CAD build for the part. Positions are in the model's coordinates, mm. Face numbers are marked on the shaded views. A direction names the side the tool comes from. Coordinates: 2 decimals unless noted, no trailing zeros. Loops run counter-clockwise (first coordinate to the right, second up) from the corner with the lowest first, then second, coordinate; pieces in that order, holes last. Notation, with made-up numbers: (-5, 57) -> (26, 57) arc R15 cw to (26, 80) -> close; hole circle Ø5 at (-14.75, 33.5). An arc over 180 degrees is marked (long way). Write each question's results on one line, items separated by ' | '.
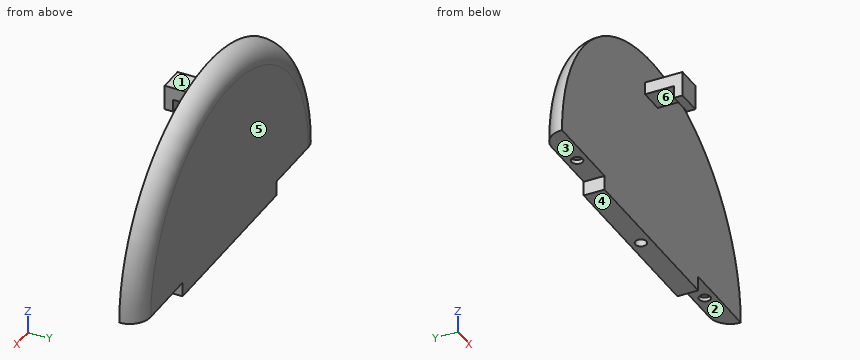
from build123d import *

# Parameters (mm, degrees)
CUT_EXTRUDE1_DEPTH       = 5
CUT_EXTRUDE3_DEPTH       = 45
SKETCH8_R                = 40
CUT_EXTRUDE4_DEPTH       = 32
SKETCH9_R                = 32
SKETCH9_R_2              = 24.5
CUT_EXTRUDE5_DEPTH       = 14
SKETCH10_R               = 26
CUT_EXTRUDE6_DEPTH       = 14
FILLET1_R                = 7
FILLET2_R                = 7
CUT_REVOLVE1_START       = 22
CUT_REVOLVE1_DEPTH       = 30.5
CUT_EXTRUDE12_DEPTH      = 5
SKETCH18_W               = 13
SKETCH18_H               = 8
CUT_EXTRUDE13_DEPTH      = 5
INTERSECT1_OUTLINE_R     = 42
INTERSECT1_DEPTH         = 55
SKETCH20_W               = 6
SKETCH20_H               = 3
BOSS_EXTRUDE1_DEPTH      = 8
BOSS_EXTRUDE2_DEPTH      = 1
BOSS_EXTRUDE2_DEPTH_BACK = 1
SKETCH21_W               = 6
SKETCH21_H               = 6
BOSS_EXTRUDE3_DEPTH      = 7
SKETCH19_R               = 1.35
CUT_EXTRUDE14_DEPTH      = 8
SKETCH23_W               = 20
SKETCH23_H               = 7
CUT_EXTRUDE15_DEPTH      = 7
SKETCH24_W               = 44
SKETCH24_H               = 3.5
CUT_EXTRUDE16_DEPTH      = 5


with BuildPart() as part:
    # Sketch1 → Revolve1 (revolve)
    with BuildSketch(Plane.XY, mode=Mode.PRIVATE) as revolve1_sk:
        with BuildLine():
            Line((22.5, 0), (32, 0))
            ThreePointArc((32, 0), (33.414213562, 0.585786438), (34, 2))
            Line((34, 2), (34, 18))
            Line((34, 18), (40, 18))
            ThreePointArc((40, 18), (41.414213562, 18.585786438), (42, 20))
            Line((42, 20), (42, 55))
            ThreePointArc((42, 55), (40.535533906, 58.535533906), (37, 60))
            Line((37, 60), (0, 60))
            Line((0, 60), (0, 18))
            Line((0, 18), (22.5, 18))
            Line((22.5, 18), (22.5, 0))
        make_face()
    revolve(revolve1_sk.sketch.rotate(Axis((0, 2, 0), (0, 1, 0)), 90), axis=Axis((0, 2, 0), (0, 1, 0)))

    # Sketch5 → Cut-Extrude1 (cut)
    with BuildSketch(Plane(origin=(0, 60, 0), x_dir=(1, 0, 0), z_dir=(0, 1, 0))):
        with BuildLine():
            Line((-42, 0), (-40, 0))
            Line((-40, 0), (40, 0))
            Line((40, 0), (42, 0))
            ThreePointArc((42, 0), (0, 42), (-42, 0))
        make_face()
    extrude(amount=-CUT_EXTRUDE1_DEPTH, mode=Mode.SUBTRACT)

    # Sketch7 → Cut-Extrude3 (cut)
    with BuildSketch(Plane.XZ.offset(-18)):
        with BuildLine():
            Line((-21, 0), (21, 0))
            ThreePointArc((21, 0), (0, -21), (-21, 0))
        make_face()
    extrude(amount=-CUT_EXTRUDE3_DEPTH, mode=Mode.SUBTRACT)

    # Sketch8 → Cut-Extrude4 (cut)
    with BuildSketch(Plane(origin=(0, 52.5, 0), x_dir=(1, 0, 0), z_dir=(0, 1, 0))):
        with Locations(Location((0, 0, 0), (0, 0, 270))):
            Circle(SKETCH8_R)
        with BuildLine():
            Line((22.912878475, -2), (-22.912878475, -2))
            ThreePointArc((-22.912878475, -2), (0, 23), (22.912878475, -2))
        make_face(mode=Mode.SUBTRACT)
    extrude(amount=-CUT_EXTRUDE4_DEPTH, mode=Mode.SUBTRACT)

    # Sketch9 → Cut-Extrude5 (cut)
    with BuildSketch(Plane(origin=(0, 2, 0), x_dir=(-1, 0, 0), z_dir=(0, -1, 0))):
        with Locations(Location((0, 0, 0), (0, 0, 90))):
            Circle(SKETCH9_R)
        with Locations(Location((0, 0, 0), (0, 0, 90))):
            Circle(SKETCH9_R_2, mode=Mode.SUBTRACT)
    extrude(amount=-CUT_EXTRUDE5_DEPTH, mode=Mode.SUBTRACT)

    # Sketch10 → Cut-Extrude6 (cut)
    with BuildSketch(Plane(origin=(0, 2, 0), x_dir=(-1, 0, 0), z_dir=(0, -1, 0))):
        Circle(SKETCH10_R)
    extrude(amount=-CUT_EXTRUDE6_DEPTH, mode=Mode.SUBTRACT)

    # Fillet1
    fillet1_edges = [part.edges().sort_by_distance(p)[0] for p in [
        (21, 36.5, 0),
        (-21, 36.5, 0),
    ]]
    fillet(fillet1_edges, radius=FILLET1_R)

    # Fillet2
    fillet2_edges = [part.edges().sort_by_distance(p)[0] for p in [
        (-22.912878475, 36.5, 2),
        (22.912878475, 36.5, 2),
    ]]
    fillet(fillet2_edges, radius=FILLET2_R)

    # Cut-Revolve1: read off the stored shape, not the designer's step
    # Cut-Revolve1 outline → Cut-Revolve1 (cut)
    with BuildSketch(Plane(origin=(0, 0, 0), x_dir=(1, 0, 0), z_dir=(0, 1, 0)).offset(CUT_REVOLVE1_START)):
        with BuildLine():
            Line((-34.641016151, -20), (-36.373066959, -21))
            ThreePointArc((-36.373066959, -21), (0, -42), (36.373066959, -21))
            Line((36.373066959, -21), (34.641016151, -20))
            ThreePointArc((34.641016151, -20), (0, -40), (-34.641016151, -20))
        make_face()
    extrude(amount=CUT_REVOLVE1_DEPTH, mode=Mode.SUBTRACT)

    # Sketch15 → Cut-Extrude12 (cut)
    with BuildSketch(Plane(origin=(0, 20.5, 0), x_dir=(1, 0, 0), z_dir=(0, 1, 0))):
        with BuildLine():
            Line((-28.124355653, -3.514579578), (-26.124355653, -3.514579578))
            ThreePointArc((-26.124355653, -3.514579578), (-24.710142091, -2.928793141), (-24.124355653, -1.514579578))
            Line((-24.124355653, -1.514579578), (-24.124355653, 8.485420422))
            ThreePointArc((-24.124355653, 8.485420422), (-24.710142091, 9.899633984), (-26.124355653, 10.485420422))
            Line((-26.124355653, 10.485420422), (-28.124355653, 10.485420422))
            ThreePointArc((-28.124355653, 10.485420422), (-29.538569215, 9.899633984), (-30.124355653, 8.485420422))
            Line((-30.124355653, 8.485420422), (-30.124355653, -1.514579578))
            ThreePointArc((-30.124355653, -1.514579578), (-29.538569215, -2.928793141), (-28.124355653, -3.514579578))
        make_face()
    extrude(amount=-CUT_EXTRUDE12_DEPTH, mode=Mode.SUBTRACT)

    # Sketch18 → Cut-Extrude13 (cut)
    with BuildSketch(Plane(origin=(0, 55, 0), x_dir=(1, 0, 0), z_dir=(0, 1, 0))):
        with Locations((0.796512215, 32.951769165)):
            Rectangle(SKETCH18_W, SKETCH18_H)
    extrude(amount=-CUT_EXTRUDE13_DEPTH, mode=Mode.SUBTRACT)

    # Intersect1: read off the stored shape, not the designer's step
    # Intersect1 outline → Intersect1 (cut)
    with BuildSketch(Plane(origin=(0, 0, 0), x_dir=(1, 0, 0), z_dir=(0, 1, 0))):
        Circle(INTERSECT1_OUTLINE_R)
        with BuildLine():
            Line((12.124355653, 0), (-12.124355653, 0))
            ThreePointArc((-12.124355653, 0), (-18.186533479, 3.5), (-18.186533479, 10.5))
            ThreePointArc((-18.186533479, 10.5), (0, 21), (18.186533479, 10.5))
            ThreePointArc((18.186533479, 10.5), (18.186533479, 3.5), (12.124355653, 0))
        make_face(mode=Mode.SUBTRACT)
    extrude(amount=INTERSECT1_DEPTH, mode=Mode.SUBTRACT)

    # Sketch20 → Boss-Extrude1 (add)
    with BuildSketch(Plane.XZ.offset(-55)):
        with Locations((0, 33.5)):
            Rectangle(SKETCH20_W, SKETCH20_H)
    extrude(amount=BOSS_EXTRUDE1_DEPTH)

    # Sketch21 → Boss-Extrude2 (add, two sides: drawn at the far end of the back side and taken through both)
    with BuildSketch(Plane.XZ.offset(-47).offset(-BOSS_EXTRUDE2_DEPTH_BACK)):
        with Locations((0, 32)):
            Rectangle(SKETCH21_W, SKETCH21_H)
    extrude(amount=BOSS_EXTRUDE2_DEPTH + BOSS_EXTRUDE2_DEPTH_BACK)

    # Sketch22 → Boss-Extrude3 (add)
    with BuildSketch(Plane(origin=(0, 0, 0), x_dir=(-1, 0, 0), z_dir=(0, 0, -1))):
        with BuildLine():
            Line((-42, 55), (42, 55))
            ThreePointArc((42, 55), (40.535533906, 58.535533906), (37, 60))
            Line((37, 60), (-37, 60))
            ThreePointArc((-37, 60), (-40.535533906, 58.535533906), (-42, 55))
        make_face()
    extrude(amount=BOSS_EXTRUDE3_DEPTH)

    # Sketch19 → Cut-Extrude14 (cut)
    with BuildSketch(Plane(origin=(0, 0, -7), x_dir=(-1, 0, 0), z_dir=(0, 0, -1))):
        with Locations((0, 57.5)):
            Circle(SKETCH19_R)
        with Locations((-30, 57.5)):
            Circle(SKETCH19_R)
        with Locations((30, 57.5)):
            Circle(SKETCH19_R)
    extrude(amount=-CUT_EXTRUDE14_DEPTH, mode=Mode.SUBTRACT)

    # Sketch23 → Cut-Extrude15 (cut)
    with BuildSketch(Plane(origin=(0, 60, 0), x_dir=(1, 0, 0), z_dir=(0, 1, 0))):
        with Locations((-32, 3.5)):
            Rectangle(SKETCH23_W, SKETCH23_H)
        with Locations((32, 3.5)):
            Rectangle(SKETCH23_W, SKETCH23_H)
    extrude(amount=-CUT_EXTRUDE15_DEPTH, mode=Mode.SUBTRACT)

    # Sketch24 → Cut-Extrude16 (cut)
    with BuildSketch(Plane(origin=(0, 60, 0), x_dir=(1, 0, 0), z_dir=(0, 1, 0))):
        with Locations((0, 5.25)):
            Rectangle(SKETCH24_W, SKETCH24_H)
    extrude(amount=-CUT_EXTRUDE16_DEPTH, mode=Mode.SUBTRACT)


solid = part.part
1) Slice it at A-A (y = 57.5). Write the cut outline in (x, z), then the cut area to 3 significant figures.
Outcome:
outline: (-41.33, 0) -> (-31.35, 0) -> (-31.35, 1) -> (-28.65, 1) -> (-28.65, 0) -> (-22, 0) -> (-22, -3.5) -> (-1.35, -3.5) -> (-1.35, 1) -> (1.35, 1) -> (1.35, -3.5) -> (22, -3.5) -> (22, 0) -> (28.65, 0) -> (28.65, 1) -> (31.35, 1) -> (31.35, 0) -> (41.33, 0) arc R41.33 ccw to start | area: 2,820 mm^2
2) Drill centre lines: L1, parallel to Y at x = -30, z = 0.3; L2, parallel to Y at x = -18, z = 25; L3, parallel to Z at x = 28, y = 56.5. Where is each one in solid material? Low to high. Write a range as from..to.
Outcome:
L1: y = 55..56.15, 58.85..60 | L2: y = 55..60 | L3: z = 0..31
3) Pin check, flat tips, straight feed: pin 1 (6.5 mm diameter, centred on y = 51.5, z = 32, fed in from -X); pin 2 (3 mm diameter, centred on x = 0, y = 49.5, fed in from +Z); pin 3 (6.5 mm diameter, centred on y = 49, z = 32, fed in from +X). Stop position of each tip, or through.
Outcome:
pin 1: stops at x = -3 | pin 2: stops at z = 35 | pin 3: stops at x = 3
4) Slice it at B-B (y = 50.5). Write the cut outline in (x, z).
Outcome:
outline: (-3, 32) -> (3, 32) -> (3, 35) -> (-3, 35) -> close
5) Two-plate mould, pull along Y, no slides. Class the marked faces 4, 5 and 6: pulls with the +Y half, pulls with the -Y half, needs draft (parallel to the pull), parting line crosses it, or undercut.
Outcome:
face 4: needs draft | face 5: pulls with the +Y half | face 6: undercut
6) Which spindle directions (+Z, -Z, +X, -X, +Y, -Y) get a long thin tool onto all of the face, cutting with end or side? Do the marked faces 1, 2 and 3. Say none if no direction does.
Outcome:
face 1: +Z, +X, -X, -Y | face 2: -Z, +X, +Y, -Y | face 3: -Z, -X, +Y, -Y
